from build123d import *

# Parameters (mm, degrees)
F1_DEPTH = 209.55
F2_W     = 69.85
F2_H     = 55.5625
F3_DEPTH = 0.4064


# Not quite as in the source:
# - the dataset's text gives a spline's control points without its knots; the knots are read off the source's solid


with BuildPart() as f1:
    # F0 (on Right) → F1 (new body, symmetric)
    with BuildSketch(Plane.YZ):
        Polygon((-139.7, 0), (0, 0), (0, 50.8), (-139.2936, 50.8), (-139.2936, 51.054), (0, 51.054), (0, 51.4604), (-139.7, 51.4604), align=None)
    extrude(amount=F1_DEPTH, both=True)

    # F2 (on face) → F3 (cut, through all)
    with BuildSketch(Plane.XY.offset(51.4604)):
        with Locations((-129.8449253923, -46.8822261976)):
            Rectangle(F2_W, F2_H)
        Polygon((108.2948828077, -19.1009761976), (38.4448828077, -19.1009761976), (38.4448828077, -74.6634761976), (108.2948828077, -74.6634761976), (108.2948828077, -68.4133743976), (108.2948828077, -42.0156877976), align=None)
        with BuildLine():
            add(Edge.make_bspline(
                [(130.8209744077, -61.8670069976), (130.3807162077, -62.3079763976), (130.1230078077, -62.9274315976), (130.1230078077, -63.5509761976)],
                knots=[1, 1, 1, 1, 2, 2, 2, 2], degree=3))
            Line((130.1230078077, -63.5509761976), (130.1230078077, -72.2822261976))
            add(Edge.make_bspline(
                [(130.1230078077, -72.2822261976), (130.1230078077, -72.9057961976), (130.3807162077, -73.5252259976), (130.8209744077, -73.9654841976)],
                knots=[0, 0, 0, 0, 1, 1, 1, 1], degree=3))
            add(Edge.make_bspline(
                [(130.8209744077, -73.9654841976), (131.2619438077, -74.4064789976), (131.8813990077, -74.6634761976), (132.5042578077, -74.6634761976)],
                knots=[1, 1, 1, 1, 2, 2, 2, 2], degree=3))
            Line((132.5042578077, -74.6634761976), (141.2355078077, -74.6634761976))
            add(Edge.make_bspline(
                [(141.2355078077, -74.6634761976), (141.8597382077, -74.6634761976), (142.4784822077, -74.4064789976), (142.9194516077, -73.9654841976)],
                knots=[0, 0, 0, 0, 1, 1, 1, 1], degree=3))
            add(Edge.make_bspline(
                [(142.9194516077, -73.9654841976), (143.3604210077, -73.5252259976), (143.6167578077, -72.9057961976), (143.6167578077, -72.2822261976)],
                knots=[1, 1, 1, 1, 2, 2, 2, 2], degree=3))
            Line((143.6167578077, -72.2822261976), (143.6167578077, -63.5509761976))
            add(Edge.make_bspline(
                [(143.6167578077, -63.5509761976), (143.6167578077, -62.9274315976), (143.3604210077, -62.3079763976), (142.9194516077, -61.8670069976), (142.4784822077, -61.4260375976), (141.8597382077, -61.1697261976), (141.2355078077, -61.1697261976)],
                knots=[0, 0, 0, 0, 1, 1, 1, 2, 2, 2, 2], degree=3))
            Line((141.2355078077, -61.1697261976), (132.5042578077, -61.1697261976))
            add(Edge.make_bspline(
                [(132.5042578077, -61.1697261976), (131.8813990077, -61.1697261976), (131.2619438077, -61.4260375976), (130.8209744077, -61.8670069976)],
                knots=[0, 0, 0, 0, 1, 1, 1, 1], degree=3))
        make_face()
        with BuildLine():
            add(Edge.make_bspline(
                [(-69.1344295923, -26.6533105976), (-70.8976467923, -24.8901187976), (-73.3763565923, -23.8634761976), (-75.8699253923, -23.8634761976)],
                knots=[7, 7, 7, 7, 8, 8, 8, 8], degree=3))
            add(Edge.make_bspline(
                [(-75.8699253923, -23.8634761976), (-78.3631639923, -23.8634761976), (-80.8419245923, -24.8901187976), (-82.6050909923, -26.6533105976), (-84.3682827923, -28.4165277976), (-85.3949253923, -30.8949327976), (-85.3949253923, -33.3884761976), (-85.3949253923, -35.8820449976), (-84.3682827923, -38.3604499976), (-82.6050909923, -40.1236163976)],
                knots=[0, 0, 0, 0, 1, 1, 1, 2, 2, 2, 3, 3, 3, 3], degree=3))
            add(Edge.make_bspline(
                [(-82.6050909923, -40.1236163976), (-80.8419245923, -41.8868589976), (-78.3631639923, -42.9134761976), (-75.8699253923, -42.9134761976), (-73.3763565923, -42.9134761976), (-70.8976467923, -41.8868589976), (-69.1344295923, -40.1236163976)],
                knots=[3, 3, 3, 3, 4, 4, 4, 5, 5, 5, 5], degree=3))
            add(Edge.make_bspline(
                [(-69.1344295923, -40.1236163976), (-67.3712377923, -38.3604499976), (-66.3449253923, -35.8820449976), (-66.3449253923, -33.3884761976), (-66.3449253923, -30.8949327976), (-67.3712377923, -28.4165277976), (-69.1344295923, -26.6533105976)],
                knots=[5, 5, 5, 5, 6, 6, 6, 7, 7, 7, 7], degree=3))
        make_face()
        with BuildLine():
            add(Edge.make_bspline(
                [(-69.1344295923, -58.4033105976), (-70.8976467923, -56.6401187976), (-73.3763565923, -55.6134761976), (-75.8699253923, -55.6134761976)],
                knots=[7, 7, 7, 7, 8, 8, 8, 8], degree=3))
            add(Edge.make_bspline(
                [(-75.8699253923, -55.6134761976), (-78.3631639923, -55.6134761976), (-80.8419245923, -56.6401187976), (-82.6050909923, -58.4033105976), (-84.3682827923, -60.1665277976), (-85.3949253923, -62.6449327976), (-85.3949253923, -65.1384761976), (-85.3949253923, -67.6320449976), (-84.3682827923, -70.1104499976), (-82.6050909923, -71.8736163976)],
                knots=[0, 0, 0, 0, 1, 1, 1, 2, 2, 2, 3, 3, 3, 3], degree=3))
            add(Edge.make_bspline(
                [(-82.6050909923, -71.8736163976), (-80.8419245923, -73.6368589976), (-78.3631639923, -74.6634761976), (-75.8699253923, -74.6634761976), (-73.3763565923, -74.6634761976), (-70.8976467923, -73.6368589976), (-69.1344295923, -71.8736163976)],
                knots=[3, 3, 3, 3, 4, 4, 4, 5, 5, 5, 5], degree=3))
            add(Edge.make_bspline(
                [(-69.1344295923, -71.8736163976), (-67.3712377923, -70.1104499976), (-66.3449253923, -67.6320449976), (-66.3449253923, -65.1384761976), (-66.3449253923, -62.6449327976), (-67.3712377923, -60.1665277976), (-69.1344295923, -58.4033105976)],
                knots=[5, 5, 5, 5, 6, 6, 6, 7, 7, 7, 7], degree=3))
        make_face()
        with BuildLine():
            add(Edge.make_bspline(
                [(-40.5442911923, -58.4033105976), (-42.3074575923, -56.6401187976), (-44.7858879923, -55.6134761976), (-47.2794567923, -55.6134761976)],
                knots=[7, 7, 7, 7, 8, 8, 8, 8], degree=3))
            add(Edge.make_bspline(
                [(-47.2794567923, -55.6134761976), (-49.7733303923, -55.6134761976), (-52.2517353923, -56.6401187976), (-54.0149271923, -58.4033105976), (-55.7781443923, -60.1665277976), (-56.8044567923, -62.6449327976), (-56.8044567923, -65.1384761976), (-56.8044567923, -67.6320449976), (-55.7781443923, -70.1104499976), (-54.0149271923, -71.8736163976)],
                knots=[0, 0, 0, 0, 1, 1, 1, 2, 2, 2, 3, 3, 3, 3], degree=3))
            add(Edge.make_bspline(
                [(-54.0149271923, -71.8736163976), (-52.2517353923, -73.6368589976), (-49.7733303923, -74.6634761976), (-47.2794567923, -74.6634761976), (-44.7858879923, -74.6634761976), (-42.3074575923, -73.6368589976), (-40.5442911923, -71.8736163976)],
                knots=[3, 3, 3, 3, 4, 4, 4, 5, 5, 5, 5], degree=3))
            add(Edge.make_bspline(
                [(-40.5442911923, -71.8736163976), (-38.7807183923, -70.1104499976), (-37.7547615923, -67.6320449976), (-37.7547615923, -65.1384761976), (-37.7547615923, -62.6449327976), (-38.7807183923, -60.1665277976), (-40.5442911923, -58.4033105976)],
                knots=[5, 5, 5, 5, 6, 6, 6, 7, 7, 7, 7], degree=3))
        make_face()
        with BuildLine():
            add(Edge.make_bspline(
                [(-40.5442911923, -26.6533105976), (-42.3074575923, -24.8901187976), (-44.7858879923, -23.8634761976), (-47.2794567923, -23.8634761976)],
                knots=[7, 7, 7, 7, 8, 8, 8, 8], degree=3))
            add(Edge.make_bspline(
                [(-47.2794567923, -23.8634761976), (-49.7733303923, -23.8634761976), (-52.2517353923, -24.8901187976), (-54.0149271923, -26.6533105976), (-55.7781443923, -28.4165277976), (-56.8044567923, -30.8949327976), (-56.8044567923, -33.3884761976), (-56.8044567923, -35.8820449976), (-55.7781443923, -38.3604499976), (-54.0149271923, -40.1236163976)],
                knots=[0, 0, 0, 0, 1, 1, 1, 2, 2, 2, 3, 3, 3, 3], degree=3))
            add(Edge.make_bspline(
                [(-54.0149271923, -40.1236163976), (-52.2517353923, -41.8868589976), (-49.7733303923, -42.9134761976), (-47.2794567923, -42.9134761976), (-44.7858879923, -42.9134761976), (-42.3074575923, -41.8868589976), (-40.5442911923, -40.1236163976)],
                knots=[3, 3, 3, 3, 4, 4, 4, 5, 5, 5, 5], degree=3))
            add(Edge.make_bspline(
                [(-40.5442911923, -40.1236163976), (-38.7807183923, -38.3604499976), (-37.7547615923, -35.8820449976), (-37.7547615923, -33.3884761976), (-37.7547615923, -30.8949327976), (-38.7807183923, -28.4165277976), (-40.5442911923, -26.6533105976)],
                knots=[5, 5, 5, 5, 6, 6, 6, 7, 7, 7, 7], degree=3))
        make_face()
        with BuildLine():
            add(Edge.make_bspline(
                [(173.3906378077, -63.1458461976), (172.1421516077, -61.8966487976), (170.3872148077, -61.1697261976), (168.6198828077, -61.1697261976)],
                knots=[7, 7, 7, 7, 8, 8, 8, 8], degree=3))
            add(Edge.make_bspline(
                [(168.6198828077, -61.1697261976), (166.8539224077, -61.1697261976), (165.0989856077, -61.8966487976), (163.8497882077, -63.1458461976)],
                knots=[0, 0, 0, 0, 1, 1, 1, 1], degree=3))
            add(Edge.make_bspline(
                [(163.8497882077, -63.1458461976), (162.6006162077, -64.3943577976), (161.8730078077, -66.1499549976), (161.8730078077, -67.9166011976), (161.8730078077, -69.6825615976), (162.6006162077, -71.4381841976), (163.8497882077, -72.6873815976)],
                knots=[1, 1, 1, 1, 2, 2, 2, 3, 3, 3, 3], degree=3))
            add(Edge.make_bspline(
                [(163.8497882077, -72.6873815976), (165.0989856077, -73.9358677976), (166.8539224077, -74.6634761976), (168.6198828077, -74.6634761976), (170.3872148077, -74.6634761976), (172.1421516077, -73.9358677976), (173.3906378077, -72.6873815976)],
                knots=[3, 3, 3, 3, 4, 4, 4, 5, 5, 5, 5], degree=3))
            add(Edge.make_bspline(
                [(173.3906378077, -72.6873815976), (174.6398098077, -71.4381841976), (175.3667578077, -69.6825615976), (175.3667578077, -67.9166011976), (175.3667578077, -66.1499549976), (174.6398098077, -64.3943577976), (173.3906378077, -63.1458461976)],
                knots=[5, 5, 5, 5, 6, 6, 6, 7, 7, 7, 7], degree=3))
        make_face()
    extrude(amount=-F3_DEPTH, mode=Mode.SUBTRACT)


solid = f1.part
For this review, take the finished solid that the model builds, in its own axes (mm). Round coordinates to 2 decimals unless told otherwise and drop trailing zeros. Write item = value, one per line. Start each with the question number.
(1) For line 1 along Z through (x, y) = (135, -114.5); line 2 along Z through (x, y) = (47, -45.5), list the stretches that pass through material, from the lowest coordinate up.
(2) The part is to be moulded in two halves that separate along Z. For faces 1 (the face through (3, -71, 51.054)), 2 (the face through (3, -69, 50.8)), 3 (the face through (3, -69, 51.46)), 4 (the face through (-209.55, -71, 26)), say which applies: +Z half, -Z half, draft (parallel to the pull), parting line (faces both ways), or undercut.
(3) Clearance check with a flat-ended pin moving along its axis: pin 1 Ø1 at (x, y) = (-106.5, -32.5) entering from +Z. State where the tip first meets the part, or that it passes through.
Results found:
q1.line_1 = 0 to 50.8, 51.05 to 51.46
q1.line_2 = 0 to 50.8
q2.face_1 = undercut
q2.face_2 = undercut
q2.face_3 = +Z half
q2.face_4 = draft
q3.pin_1 = 50.8
